Autodesk Inventor part; units mm, degrees
ref_plane "YZ Plane" through (0, 0, 0) normal (1, 0, 0) x (0, 1, 0)
ref_plane "XZ Plane" through (0, 0, 0) normal (0, 1, 0) x (-1, 0, 0)
ref_plane "XY Plane" through (0, 0, 0) normal (0, 0, 1) x (1, 0, 0)
sketch "profile_sketch" plane through (0, 0, 0) normal (0, 0, 1) x (1, 0, 0)
  line L0 (0, 0) -> (25.4, 0)
  line L1 (25.4, 0) -> (25.4, 25.4)
  line L2 (25.4, 25.4) -> (0, 25.4)
  line L3 (0, 25.4) -> (0, 0)
  line L4 (1.5875, 23.8125) -> (23.8125, 23.8125)
  line L5 (23.8125, 23.8125) -> (23.8125, 1.5875)
  line L6 (23.8125, 1.5875) -> (1.5875, 1.5875)
  line L7 (1.5875, 1.5875) -> (1.5875, 23.8125)
  dimension "d0" = 25.4
  dimension "d1" = 25.4
  dimension "d2" = 1.5875
  dimension "d3" = 1.5875
  dimension "d4" = 1.5875
  dimension "d5" = 1.5875
extrude "profile_extrusion" add sketch "profile_sketch" along normal blind 685.8
sketch "gbmh_sketch" plane through (25.4, 0, 0) normal (1, 0, 0) x (0, 0, -1)
  line L0 (-685.8, 0) -> (-685.8, 25.4) construction
  line L1 (-685.8, 12.7) -> (-342.9, 12.7) construction
  line L2 (-342.9, 12.7) -> (0, 12.7) construction
  line L3 (0, 25.4) -> (0, 0) construction
  line L4 (-342.9, 12.7) -> (-342.9, 25.4) construction
  line L5 (0, 25.4) -> (-685.8, 25.4) construction
  line L6 (-342.9, 12.7) -> (-342.9, 0) construction
  point P0 (-398.4752, 12.7)
  point P1 (-287.3248, 12.7)
  dimension "d8" = 55.5752
hole "gbmh" at (25.4, 12.7, 398.4752) at (25.4, 12.7, 287.3248) direction (-1, 0, 0) diameter 6.35 depth 25.4 tip angle 118
sketch "side_rivet_holes_sketch" plane through (0, 0, 0) normal (-1, 0, 0) x (0, 0, 1)
  line L0 (0, 25.4) -> (0, 0) construction
  line L1 (0, 12.7) -> (342.9, 12.7) construction
  line L2 (0, 1.5875) -> (685.8, 1.5875) construction
  line L3 (342.9, 12.7) -> (685.8, 12.7) construction
  line L4 (685.8, 25.4) -> (685.8, 0) construction
  line L5 (342.9, 12.7) -> (342.9, 25.4) construction
  line L6 (342.9, 12.7) -> (342.9, 0) construction
  line L7 (0, 0) -> (685.8, 0) construction
  point P0 (19.05, 12.7)
  point P1 (38.1, 12.7)
  point P2 (57.15, 12.7)
  point P3 (628.65, 12.7)
  point P4 (647.7, 12.7)
  point P5 (666.75, 12.7)
  dimension "d21" = 19.05
  dimension "d22" = 19.05
  dimension "d35" = 19.05
  dimension "d36" = 19.05
  dimension "d45" = 19.05
  dimension "d46" = 19.05
hole "side_rivet_holes" at (0, 12.7, 19.05) at (0, 12.7, 38.1) at (0, 12.7, 57.15) at (0, 12.7, 628.65) at (0, 12.7, 647.7) at (0, 12.7, 666.75) direction (1, 0, 0) diameter 3.5719 depth 25.4 tip angle 118
sketch "crossbar_rivet_holes_sketch" plane through (0, 25.4, 0) normal (0, 1, 0) x (1, 0, 0)
  line L0 (0, 0) -> (0, -685.8)
  line L1 (25.4, 0) -> (25.4, -685.8)
  line L2 (25.4, -139.7) -> (0, -139.7) construction
  line L3 (25.4, -266.7) -> (0, -266.7) construction
  line L4 (25.4, -419.1) -> (0, -419.1) construction
  line L5 (0, 0) -> (0, -685.8)
  line L6 (25.4, -546.1) -> (0, -546.1) construction
  line L7 (25.4, 0) -> (0, 0)
  line L8 (25.4, -685.8) -> (0, -685.8)
  line L9 (12.7, -139.7) -> (12.7, -160.8667) construction
  line L10 (12.7, -160.8667) -> (12.7, -182.0333) construction
  line L11 (12.7, -182.0333) -> (12.7, -203.2) construction
  line L12 (12.7, -203.2) -> (12.7, -224.3667) construction
  line L13 (12.7, -224.3667) -> (12.7, -245.5333) construction
  line L14 (12.7, -245.5333) -> (12.7, -266.7) construction
  line L15 (12.7, -419.1) -> (12.7, -440.2667) construction
  line L16 (12.7, -440.2667) -> (12.7, -461.4333) construction
  line L17 (12.7, -461.4333) -> (12.7, -482.6) construction
  line L18 (12.7, -482.6) -> (12.7, -503.7667) construction
  line L19 (12.7, -503.7667) -> (12.7, -524.9333) construction
  line L20 (12.7, -524.9333) -> (12.7, -546.1) construction
  dimension "d48" = 127
  dimension "d49" = 127
  dimension "d52" = 203.2
  dimension "d53" = 203.2
hole "tb_rivet_holes" at (12.7, 25.4, 160.8667) at (12.7, 25.4, 182.0333) at (12.7, 25.4, 203.2) at (12.7, 25.4, 224.3667) at (12.7, 25.4, 245.5333) at (12.7, 25.4, 440.2667) at (12.7, 25.4, 461.4333) at (12.7, 25.4, 482.6) at (12.7, 25.4, 503.7667) at (12.7, 25.4, 524.9333) direction (0, -1, 0) diameter 3.5719 depth 25.4 tip angle 118
equation "\"d0\" = st_outer_diameter"
equation "\"d1\" = st_outer_diameter"
equation "\"d2\" = st_wall_thickness"
equation "\"d3\" = st_wall_thickness"
equation "\"d4\" = st_wall_thickness"
equation "\"d5\" = st_wall_thickness"
equation "\"d6\" = st_length"
equation "\"d14\" = gb_mh_diameter"
equation "\"d38\" = rv_hole_diameter"
equation "\"d48\" = tb_rivet_row_length"
equation "\"d49\" = tb_rivet_row_length"
equation "\"d54\" = rv_hole_diameter"
equation "\"gb_mh_seperation\" = 111.1504"
equation "\"st_outer_diameter\" = 25.4"
equation "\"st_inner_diameter\" = 6.35"
equation "\"st_wall_thickness\" = 1.5875"
equation "\"st_length\" = 685.8"
equation "\"st_gbmh_from_center\" = 0.5 * gb_mh_seperation"
equation "\"st_cutout_depth\" = 254"
equation "\"st_rivet_distance\" = 19.05"
equation "\"gb_mh_diameter\" = 6.35"
equation "\"rv_hole_diameter\" = 3.57187"
equation "\"st_cutout_depth_right\" = 203.2"
equation "\"st_cutout_depth_left\" = 203.2"
equation "\"gb_width\" = 127"
equation "\"gb_axle_from_edge\" = 38.1"
equation "\"gb_bearing_diameter\" = 28.575"
equation "\"gb_to_bottom_of_side_assembly\" = 4.7752"
equation "\"tb_rivet_row_length\" = 127"
equation "\"tb_metal_thickness\" = 3.048"
equation "\"tb_hm_mounting_slot_length\" = 40.64"
equation "\"gb_mh_seperation_alt\" = 111.125"
equation "\"gb_axle_from_edge_alt\" = 43.1546"
properties part number "sidetube(st" material "Aluminum 6061"
Input: part model. Units: mm. Frame: model coordinates. A direction names the side the tool comes from. Give positions to 0.01 mm unless a question says otherwise; leave off trailing zeros. Order: outer loops, then holes, each group sorted by start corner. A loop starts at its lowest first (then second) coordinate and runs counter-clockwise, first axis right, second up. Notation, with made-up numbers: (55.5, 56) -> (66.5, 56) arc R17 cw to (66.5, 68) -> close; hole circle Ø1 at (42, -24.5). An arc over 180 degrees is marked (long way). Write each question's results on one line, items separated by ' | '. Start each with the question number.
Item 1: Mould query, pull axis Y, two halves, no side actions, for faces 3 (the flat face through (13, 0, 338)), 4 (the flat face through (25.4, 13, 338)), 5 (the flat face through (13, 1.588, 338)). Classes: pulls with the +Y half, pulls with the -Y half, needs draft (parallel to the pull), parting line crosses it, or undercut.
Item 2: Line query: line 1 (X direction, y = 13.5, z = 509); line 2 (Y direction, x = 1.25, z = 647.7). Output: solid intervals per line, ascending.
Item 3: Contact query for a flat-ended pin moving along its axis: P1, Ø3, axis at x = 12.7, z = 203.2, coming from the -Y side. Output: stop coordinate, or through.
Item 4: Cut plane B-B on z = 271.5. Return the cut outline in (x, y), then the cut area to 3 significant figures.
Item 5: Set-up query: faces 1 (the flat face through (0, 13, 338)), 2 (the flat face through (1.588, 13, 338)). Return all of +Z, -Z, +X, -X, +Y, -Y with unobstructed straight access to the full face (end or side cutting, diameter ignored); none if empty.
Item 6: Cut plane A-A on x = 5.5. Return the cut outline in (y, z), then the cut area to 3 significant figures.
Established:
1) face 3: pulls with the -Y half | face 4: needs draft | face 5: undercut
2) line 1: 0 to 1.59, 23.81 to 25.4 | line 2: 0 to 10.91, 14.49 to 25.4
3) P1: through
4) outline: (0, 0) -> (25.4, 0) -> (25.4, 25.4) -> (0, 25.4) -> close; hole (1.59, 1.59) -> (23.81, 1.59) -> (23.81, 23.81) -> (1.59, 23.81) -> close | area: 151 mm^2
5) face 1: +Z, -Z, -X, +Y, -Y | face 2: +Z, -Z
6) outline: (0, 0) -> (1.59, 0) -> (1.59, 685.8) -> (0, 685.8) -> close; (23.81, 0) -> (25.4, 0) -> (25.4, 685.8) -> (23.81, 685.8) -> close | area: 2,180 mm^2
